Input: dimensioned drawing with shaded views. Units: mm. Origin: part minimum x, y, z. Coordinates: 2 decimals unless noted, no trailing zeros. Order: outer loops, then holes, each group sorted by start corner. A loop starts at its lowest first (then second) coordinate and runs counter-clockwise, first axis right, second up. Notation, with made-up numbers: (-24.5, 3.5) -> (16.5, 3.5) arc R13 cw to (16.5, 25.5) -> close; hole circle Ø10 at (79, 76.25). An arc over 180 degrees is marked (long way). Answer in a Markdown table with one row per item. Add a question column.
1) Ray query, line 1 (Z direction, x = 22.87, y = 0.35); line 2 (X direction, y = 0.15, z = 11.5) (1 decimal); line 3 (X direction, y = 1, z = 12). Return the intervals inside material, ascending. Write a range as from..to.
2) Section query B-B on z = 13. Return the cut outline in (x, y).
3) Section query A-A on x = 22.87. Return the cut outline in (y, z), then the cut area to 3 significant figures.
4) Section query D-D on x = 2.55. Return the cut outline in (y, z) (1 decimal).
5) Section query C-C on y = 0.5. Return the cut outline in (x, z), then the cut area to 3 significant figures.
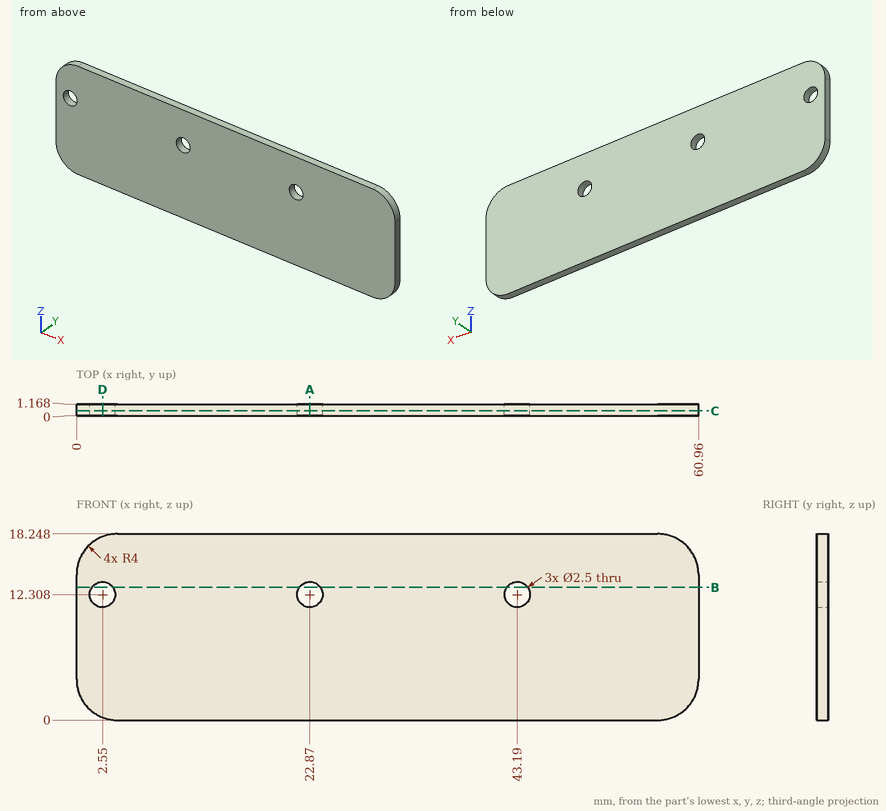
Result:
| question | item | result |
|---|---|---|
| 1 | line 1 | 0..11.06, 13.56..18.25 |
| 1 | line 2 | 0..1.6, 3.5..21.9, 23.8..42.2, 44.1..61 |
| 1 | line 3 | 0..1.34, 3.76..21.66, 24.08..41.98, 44.4..60.96 |
| 2 | outline | (0, 0) -> (1.51, 0) -> (1.51, 1.17) -> (0, 1.17) -> close; (3.59, 0) -> (21.83, 0) -> (21.83, 1.17) -> (3.59, 1.17) -> close; (23.91, 0) -> (42.15, 0) -> (42.15, 1.17) -> (23.91, 1.17) -> close; (44.23, 0) -> (60.96, 0) -> (60.96, 1.17) -> (44.23, 1.17) -> close |
| 3 | outline | (0, 0) -> (1.17, 0) -> (1.17, 11.06) -> (0, 11.06) -> close; (0, 13.56) -> (1.17, 13.56) -> (1.17, 18.25) -> (0, 18.25) -> close |
| 3 | area | 18.4 mm2 |
| 4 | outline | (0, 0.3) -> (1.2, 0.3) -> (1.2, 11.1) -> (0, 11.1) -> close; (0, 13.6) -> (1.2, 13.6) -> (1.2, 18) -> (0, 18) -> close |
| 5 | outline | (0, 4) arc R4 ccw to (4, 0) -> (56.96, 0) arc R4 ccw to (60.96, 4) -> (60.96, 14.25) arc R4 ccw to (56.96, 18.25) -> (4, 18.25) arc R4 ccw to (0, 14.25) -> close; hole circle Ø2.5 at (2.55, 12.31); hole circle Ø2.5 at (22.87, 12.31); hole circle Ø2.5 at (43.19, 12.31) |
| 5 | area | 1,080 mm2 |
